Part model, mm, in its own coordinate system. A direction names the side the tool comes from. Round coordinates to 2 decimals unless told otherwise and drop trailing zeros. Loops run counter-clockwise (first coordinate to the right, second up) from the corner with the lowest first, then second, coordinate; pieces in that order, holes last. Notation, with made-up numbers: M -18,-26.5 L 39,-26.5 A34 cw 39,5.5 Z; hole C -40,57 d10. An arc over 180 degrees is marked long. Write each question's results on one line, items separated by ' | '.
from build123d import *

# Parameters (mm, degrees)
ESQUISSE2_W                  = 149.999998509
ESQUISSE2_H                  = 85.999999195
ESQUISSE2_R                  = 1.549998298
ESQUISSE2_R_2                = 1.550002024
ESQUISSE2_R_3                = 1.550000161
BOSS_EXTRU_1_DEPTH           = 7
ENL_V_MAT_EXTRU_1_DEPTH      = 98.270805324
ENL_V_MAT_EXTRU_1_DEPTH_BACK = 98.270805324
ESQUISSE1_R                  = 2.199999988
ESQUISSE1_R_2                = 2.199999813
ESQUISSE3_W                  = 166.207428958
ESQUISSE3_H                  = 65.702519239
ENL_V_MAT_EXTRU_2_DEPTH      = 97.379507271
CONG_1_R                     = 4


with BuildPart() as part:
    # Esquisse2 → Boss.-Extru.1 (new body)
    with BuildSketch(Plane.XY):
        with Locations((0.099997967, 16.999999062)):
            Rectangle(ESQUISSE2_W, ESQUISSE2_H)
        with Locations((-69.500004873, 54.500000551)):
            Circle(ESQUISSE2_R, mode=Mode.SUBTRACT)
        with Locations((69.399992004, 54.399998859)):
            Circle(ESQUISSE2_R_2, mode=Mode.SUBTRACT)
        with Locations((69.399993867, -10.199999437)):
            Circle(ESQUISSE2_R_3, mode=Mode.SUBTRACT)
        with Locations((-45.399997383, -20.400000736)):
            Circle(ESQUISSE2_R_3, mode=Mode.SUBTRACT)
    extrude(amount=BOSS_EXTRU_1_DEPTH)

    # Esquisse1 → Enlèv. mat.-Extru.1 (cut, two sides: drawn at the far end of the back side and taken through both)
    with BuildSketch(Plane(origin=(-8.3999997, 23.400000297, 0), x_dir=(0, -1, 0), z_dir=(0, 0, 1)).offset(-ENL_V_MAT_EXTRU_1_DEPTH_BACK)):
        with Locations(Location((-30.09999916, 13.199999928, 0), (0, 0, 90))):
            Circle(ESQUISSE1_R)
        with Locations(Location((41.29999876, 41.29999876, 0), (0, 0, 90))):
            Circle(ESQUISSE1_R)
        with Locations(Location((41.899997916, -3.499999817, 0), (0, 0, 90))):
            Circle(ESQUISSE1_R_2)
        Polygon((36.100000143, 41.799999774), (32.099999487, 45.800000429), (-33.099997789, 45.800000429), (-33.099997789, 21.799998358), (-26.100000367, 14.800000004), (-26.100000367, 9.999999776), (-31.100001053, 4.999999755), (-31.100001053, -14.000000432), (34.099999815, -14.000000432), (38.099996746, -9.999999776), (38.099996746, -2.000000095), (40.099997073, 0), (48.099998385, 4.00000019), (48.099998385, 32.800000161), (44.099997729, 36.800000817), (39.099998772, 36.800000817), (36.100000143, 39.799999446), align=None)
    extrude(amount=ENL_V_MAT_EXTRU_1_DEPTH + ENL_V_MAT_EXTRU_1_DEPTH_BACK, mode=Mode.SUBTRACT)

    # Esquisse3 → Enlèv. mat.-Extru.2 (cut, through all)
    with BuildSketch(Plane.XY):
        with Locations((8.203713192, 90.85813109)):
            Rectangle(ESQUISSE3_W, ESQUISSE3_H)
    extrude(amount=ENL_V_MAT_EXTRU_2_DEPTH, mode=Mode.SUBTRACT)

    # Congé1
    cong_1_edges = [part.edges().sort_by_distance(p)[0] for p in [
        (75.099997222, 58.00687147, 3.5),
        (-74.900001287, 58.00687147, 3.5),
        (75.099997222, -26.000000536, 3.5),
        (-74.900001287, -26.000000536, 3.5),
    ]]
    fillet(cong_1_edges, radius=CONG_1_R)


solid = part.part
Item 1: Wall check: L1, parallel to Y at x = 32.9, z = 2.75; L2, parallel to Y at x = -11.9, z = 5.5; L3, parallel to X at y = 41.5, z = 6.5. Give the ranges that are in metal, low to high.
Filled sheet:
L1: -26 to -20.1, -15.7 to -12.7, 56.5 to 58.01 | L2: -26 to -20.7, -16.3 to -14.7, 54.5 to 58.01 | L3: -74.9 to -22.4, 37.4 to 75.1
Item 2: Band-saw the part on B-B on y = -3.5. Give the cut face in (x, z), and give its area (3 significant figures).
Filled sheet:
outline: M -74.9,0 L -22.4,0 L -22.4,7 L -74.9,7 Z; M 37.4,0 L 75.1,0 L 75.1,7 L 37.4,7 Z | area: 631 mm^2
Item 3: Band-saw the part on C-C on x = 4.8. Give the cut face in (y, z), and give its area (3 significant figures).
Filled sheet:
outline: M -26,0 L -24.7,0 L -24.7,7 L -26,7 Z; M 49.5,0 L 51.3,0 L 51.3,7 L 49.5,7 Z; M 55.7,0 L 58.01,0 L 58.01,7 L 55.7,7 Z | area: 37.8 mm^2
Item 4: Two-plate mould, pull along Y, no slides. Class faces 3 (the flat face through (75.1, 15, 3)), 4 (the flat face through (-1, 58.007, 3)), 5 (the cylindrical face through (30.702, -17.803, 3.451)), 6 (the flat face through (-20.4, -12.7, 3.5)): +Y half, -Y half, draft (parallel to the pull), parting line (faces both ways), or undercut.
Filled sheet:
face 3: draft | face 4: +Y half | face 5: undercut | face 6: undercut
Item 5: Band-saw the part on D-D on z = 4.75. Count the separate pieces of the cut face and the enclosed holes in it, and give its area (3 significant figures).
Filled sheet:
separate pieces: 1 | enclosed holes: 8 | area: 8,060 mm^2
Item 6: Which spindle directions (+Z, -Z, +X, -X, +Y, -Y) get a long thin tool onto all of the face, cutting with end or side? Do faces 1 (the flat face through (4, 49.5, 3)), 2 (the flat face through (-1, -26, 3)). Say none if no direction does.
Filled sheet:
face 1: +Z, -Z | face 2: +Z, -Z, +X, -X, -Y
Item 7: Drop a flat-ended pin along its axis: P1, Ø1.9, axis at x = -69.5, y = 54.5, coming from the +Z side. Give the stop position or say it passes through.
Filled sheet:
P1: through
Item 8: Band-saw the part on A-A on x = -15.5. Give the cut face in (y, z).
Filled sheet:
outline: M -26,0 L -14.7,0 L -14.7,7 L -26,7 Z; M 54.5,0 L 58.01,0 L 58.01,7 L 54.5,7 Z
